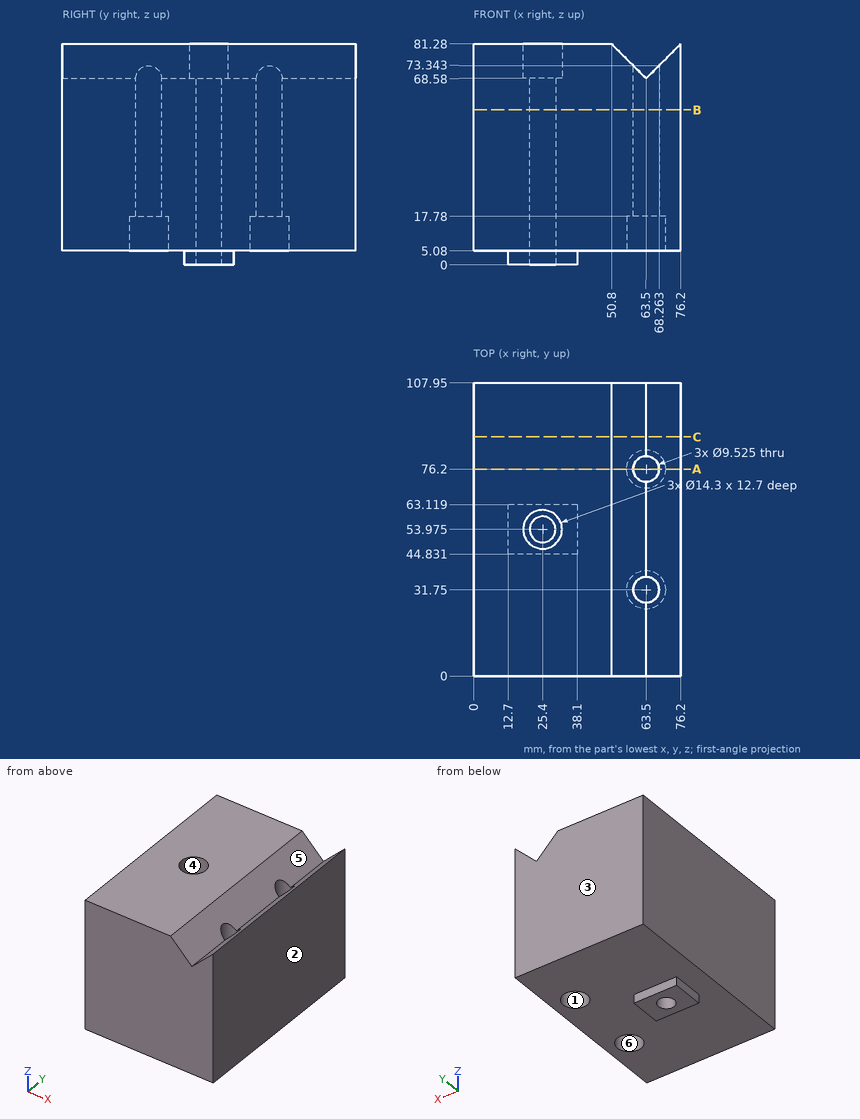
Check sheet for the drawn part. Datum: minimum x, y, z corner. Units: mm. A direction names the side the tool comes from. Round coordinates to 2 decimals unless told otherwise and drop trailing zeros. Write each loop counter-clockwise with the first axis right and the second up, starting at its lowest first coordinate (ties: lowest second). Pieces come first, ordered by that corner, then holes. Notation, with made-up numbers: (-10.75, 24) - (8.25, 24) arc R30 cw to (8.25, 54) - close; hole circle Ø5 at (84, 4). An arc over 180 degrees is marked (long way). Write each question's results on one line, items separated by ' | '.
(1) Thickness scan on probe 1 along Y at (x, z) = (63.5, 36); probe 2 along Y at (x, z) = (63.5, 13.25); probe 3 along Y at (x, z) = (25.4, 55.5). Record the ranges inside material, lowest first. Write a range as from..to.
Computed:
probe 1: y = 0..26.99, 36.51..71.44, 80.96..107.95 | probe 2: y = 0..24.6, 38.9..69.05, 83.35..107.95 | probe 3: y = 0..49.21, 58.74..107.95
(2) Depth check by flat-ended pin: pin 1 Ø8.5 at (x, y) = (63.5, 31.75) entering from +Z; pin 2 Ø4 at (y, z) = (58.5, 2.5) entering from -X; pin 3 Ø11.5 at (x, y) = (63.5, 76.2) entering from +Z; pin 4 Ø2.5 at (x, z) = (28.5, 3.5) entering from +Y. Enter the tip coordinate at first touch or a pass-through.
Computed:
pin 1: passes through | pin 2: stops at x = 12.7 | pin 3: stops at z = 74.33 | pin 4: stops at y = 63.12
(3) Set-up check for the marked faces 4, 5 and 6: record each of +Z, -Z, +X, -X, +Y, -Y from which the full face is reachable in a straight line by a thin tool's end or side.
Computed:
face 4: +Z | face 5: +Z, +Y, -Y | face 6: -Z
(4) Sectioned sample at C-C, the plane y = 88. Enter the section's corners in (x, z).
Computed:
outline: (0, 5.08) - (76.2, 5.08) - (76.2, 81.28) - (63.5, 68.58) - (50.8, 81.28) - (0, 81.28) - close
(5) Sectioned sample at A-A, the plane y = 76.2. Enter the section's corners in (x, z).
Computed:
outline: (0, 5.08) - (56.35, 5.08) - (56.35, 17.78) - (58.74, 17.78) - (58.74, 73.34) - (50.8, 81.28) - (0, 81.28) - close; (68.26, 17.78) - (70.65, 17.78) - (70.65, 5.08) - (76.2, 5.08) - (76.2, 81.28) - (68.26, 73.34) - close
(6) Draft check along Y on the marked faces 1, 2 and 3. Enter one of: pulls with the +Y half, pulls with the -Y half, needs draft (parallel to the pull), parting line crosses it, or undercut.
Computed:
face 1: undercut | face 2: needs draft | face 3: pulls with the +Y half
(7) Sectioned sample at B-B, the plane z = 57. Count the separate pieces of the cut face and the enclosed holes in it, plus the area to 3 significant figures.
Computed:
separate pieces: 1 | enclosed holes: 3 | area: 8,010 mm^2
